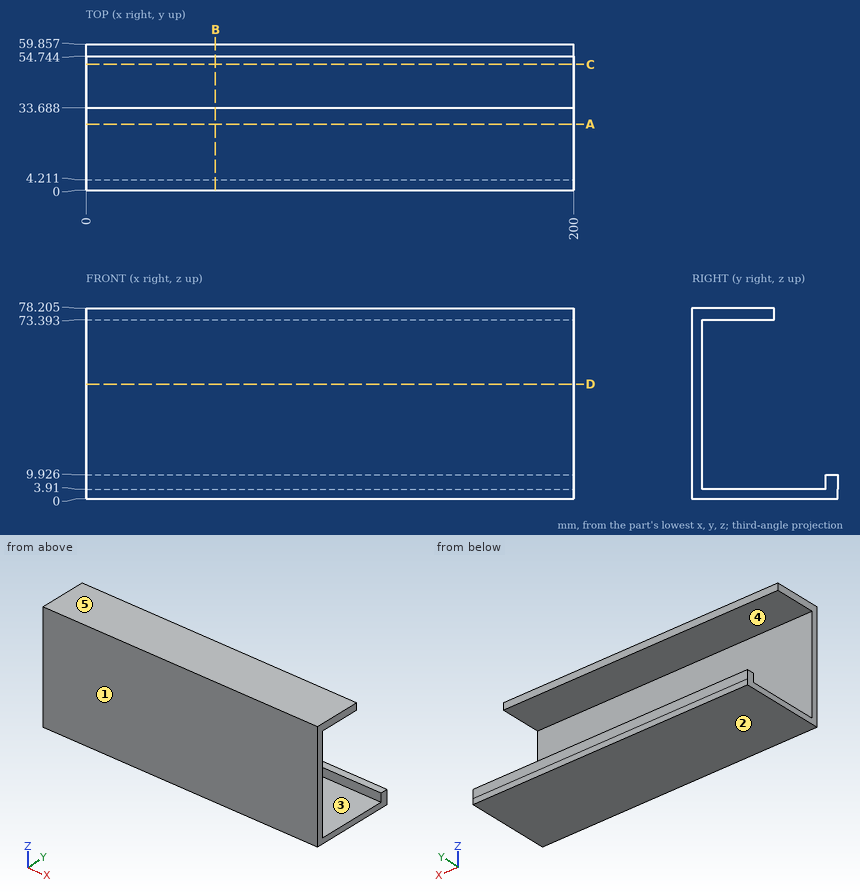
Answer from the drawing. Dimensions are ordinates in mm from the lowest x, y and z of the part. A direction names the side the tool comes from. Coordinates: 2 decimals unless noted, no trailing zeros. Write each loop counter-clockwise with the first axis right and the second up, starting at its lowest first coordinate (ties: lowest second). Pieces come first, ordered by that corner, then holes. Notation, with made-up numbers: (17, 13) - (67, 13) arc R5 ccw to (67, 22) - close; hole circle Ø11 at (59, 88.5). An arc over 180 degrees is marked (long way). One line per question, with ' | ' between items.
Q1. Find section B-B, the plane x = 53. Write down the section's boundary in (y, z) (1 decimal).
Result set:
outline: (0, 0) - (59.9, 0) - (59.9, 9.9) - (54.7, 9.9) - (54.7, 3.9) - (4.2, 3.9) - (4.2, 73.4) - (33.7, 73.4) - (33.7, 78.2) - (0, 78.2) - close
Q2. Each of these flat-tipped pins is pushed along its axis until it touches: P1, Ø4, axis at x = 142.5, z = 75.5, coming from the +Y side; P2, Ø1.5, axis at x = 66.5, y = 56.5, coming from the +Z side; P3, Ø1.5, axis at x = 30, z = 27.5, coming from the -Y side; P4, Ø2, axis at x = 127.5, z = 19, coming from the +Y side. Where does it stop, or does it pass through?
Result set:
P1: y = 33.69 | P2: z = 9.93 | P3: y = 0 | P4: y = 4.21
Q3. Find section A-A, the plane y = 27. Write down the section's boundary in (x, z) (1 decimal).
Result set:
outline: (0, 0) - (200, 0) - (200, 3.9) - (0, 3.9) - close; (0, 73.4) - (200, 73.4) - (200, 78.2) - (0, 78.2) - close
Q4. Determine the mould class of the marked faces 1, 2 and 3 for opening direction Y: +Y half, -Y half, draft (parallel to the pull), parting line (faces both ways), or undercut.
Result set:
face 1: -Y half | face 2: draft | face 3: undercut
Q5. Find section D-D, the plane z = 47. Write down the section's boundary in (x, y).
Result set:
outline: (0, 0) - (200, 0) - (200, 4.21) - (0, 4.21) - close
Q6. Find section C-C, the plane y = 51.5. Write down the section's boundary in (x, z), plus the area to 3 significant figures.
Result set:
outline: (0, 0) - (200, 0) - (200, 3.91) - (0, 3.91) - close | area: 782 mm^2
Q7. Consider L1, parallel to Z at x = 142, y = 26.5 (1 decimal); L2, parallel to Y at x = 58, z = 7.5; L3, parallel to Y at x = 134, z = 56.5. Determine where each line is inside the solid, lowest interval first. Write a range as [from, to].
Result set:
L1: [0, 3.9], [73.4, 78.2] | L2: [0, 4.21], [54.74, 59.86] | L3: [0, 4.21]
Q8. For the marked faces 4 and 5, determine the directions among +Z, -Z, +X, -X, +Y, -Y from which every point of the face is accessible in a straight line to the end or side of a thin tool.
Result set:
face 4: +X, -X, +Y | face 5: +Z, +X, -X, +Y, -Y
